Verification items for this drawing (mm, ordinates from the low corner). Coordinates: 2 decimals unless noted, no trailing zeros. Write each loop counter-clockwise with the first axis right and the second up, starting at its lowest first coordinate (ties: lowest second). Pieces come first, ordered by that corner, then holes. Notation, with made-up numbers: (31.25, 43.25) -> (84.25, 43.25) arc R20 ccw to (84.25, 56.25) -> close; hole circle Ø5 at (28.5, -14). An arc over 180 degrees is marked (long way). One line per item, written item: value. Start each with the question number.
1) Sectioned sample at A-A on y = 15. Enter the section's corners in (x, z), plus the area to 3 significant figures.
2) Gauge pin test, flat ends, axial feed: P1, Ø6, axis at y = 15, z = 20, coming from the -X side; P2, Ø3, axis at x = 6, z = 5, coming from the +Y side. Record the tip position at first contact, or that the pin passes through.
3) Scan lines: line 1 along Z through (x, y) = (6, 89.75); line 2 along Z through (x, y) = (3.5, 17); line 3 along Y through (x, z) = (3, 18). Record each from-to range of solid material in increasing order. Write a range as [from, to].
4) Sectioned sample at B-B on z = 20. Enter the section's corners in (x, y), plus the area to 3 significant figures.
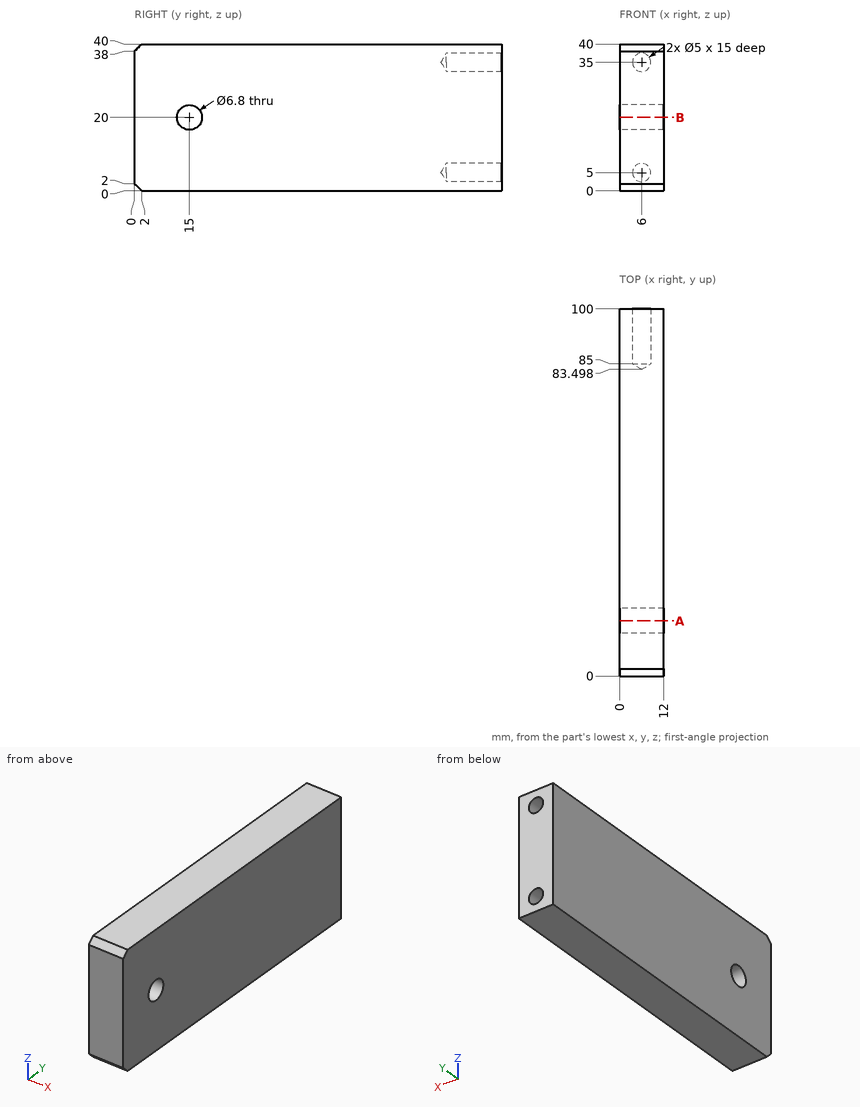
Answers:
1. outline: (0, 0) -> (12, 0) -> (12, 16.6) -> (0, 16.6) -> close; (0, 23.4) -> (12, 23.4) -> (12, 40) -> (0, 40) -> close
1. area: 398 mm2
2. P1: passes through
2. P2: stops at y = 84.4
3. line 1: z = [0, 2.5], [7.5, 32.5], [37.5, 40]
3. line 2: z = [0, 17.25], [22.75, 40]
3. line 3: y = [0, 12.25], [17.75, 100]
4. outline: (0, 0) -> (12, 0) -> (12, 11.6) -> (0, 11.6) -> close; (0, 18.4) -> (12, 18.4) -> (12, 100) -> (0, 100) -> close
4. area: 1,120 mm2
